Could you check a few things on this model? Use its own coordinates, in mm. A direction names the side the tool comes from. Coordinates: 2 decimals unless noted, no trailing zeros. Write each loop counter-clockwise with the first axis right and the second up, starting at its lowest first coordinate (ties: lowest second). Pieces come first, ordered by that corner, then holes. Notation, with made-up numbers: (31, -32.75) - (44, -32.75) arc R23 cw to (44, -16.75) - close; hole circle Ø1 at (8.25, 68.25). An arc over 180 degrees is marked (long way). Answer as a JSON object with one key per item and string values. Group by question number.
1) We'd pull the mould along Y, two halves only. Please class faces 5 (the cylindrical face through (-34.09, -12.08, 10.34)), 6 (the flat face through (-12.7, 0, 5)), 7 (the flat face through (13.36, 18.39, -13.38)): released by +Y, released by -Y, zero draft, split by the parting line, or undercut.
2) If we section it at B-B (x = -31.75): Write out the boundary of the cut face in (y, z).
3) If we section it at D-D (y = -19.5): Write out the boundary of the cut face in (x, z), plus the area to 3 significant figures.
4) Will these pins go through, and if not, where does the flat tip stop? pin 1 Ø1.5 at (y, z) = (-7.5, 12.5) entering from +X; pin 2 Ø15 at (x, y) = (12.5, 8.5) entering from +Z; pin 3 Ø12.5 at (y, z) = (-6, -9.5) entering from -X.
5) If we section it at C-C (z = 5): Write out the boundary of the cut face in (x, y), plus the area to 3 significant figures.
6) On a 3-axis mill with a long thin cutter (end or side, diameter ignored), from which of +Z, -Z, +X, -X, +Y, -Y can I reach the whole of each face in a straight line? I mean faces 1 (the flat face through (-22.098, 0, -7)), 2 (the cylindrical face through (-28.82, -19.858, 16.671)), 3 (the flat face through (-46, 0, -1.524)), 4 (the flat face through (29, -11.176, -13)). Say none if no direction works.
7) Please list where these lines run through material, in increasing order: line 1 along Y through (x, z) = (-31.75, 8.5); line 2 along Y through (x, z) = (38.1, -10.5); line 3 along X through (y, z) = (-12, 6).
8) If we section it at A-A (y = 0): Write out the boundary of the cut face in (x, z), plus the area to 3 significant figures.
```python
from build123d import *

# Parameters (mm, degrees)
F0_W     = 50.8
F0_H     = 38.1
F1_DEPTH = 50.8
F2_R     = 3.175
F3_DEPTH = 38.101
F4_W     = 63.5
F4_H     = 26.924
F5_DEPTH = 50.801
F6_R     = 6.35
F7_DEPTH = 11.177
F8_R     = 6.35
F9_DEPTH = 4.826


with BuildPart() as f1:
    # F0 (on Right) → F1 (new body, symmetric)
    with BuildSketch(Plane.YZ):
        Rectangle(F0_W, F0_H)
    extrude(amount=F1_DEPTH, both=True)

    # F2 (on face) → F3 (cut, through all)
    with BuildSketch(Plane.XY.offset(19.05)):
        with Locations((-31.75, -14.224)):
            Circle(F2_R)
        with Locations((-31.75, 14.224)):
            Circle(F2_R)
    extrude(amount=-F3_DEPTH, mode=Mode.SUBTRACT)

    # F4 (on face) → F5 (cut, through all)
    with BuildSketch(Plane.XZ.offset(25.4)):
        Polygon((-41.148, -1.524), (-50.8, -1.524), (-50.8, -19.05), (-22.098, -19.05), (-22.098, 6.35), (-41.148, 6.35), align=None)
        with Locations((19.05, 5.588)):
            Rectangle(F4_W, F4_H)
    extrude(amount=-F5_DEPTH, mode=Mode.SUBTRACT)

    # F6 (on face) → F7 (cut, through all)
    with BuildSketch(Plane.XY.offset(-7.874)):
        with BuildLine():
            ThreePointArc((38.1, 11.176), (49.276, 0), (38.1, -11.176))
            Line((38.1, -11.176), (20.574, -11.176))
            Line((20.574, -11.176), (6.35, -25.4))
            Line((6.35, -25.4), (50.8, -25.4))
            Line((50.8, -25.4), (50.8, 25.4))
            Line((50.8, 25.4), (6.35, 25.4))
            Line((6.35, 25.4), (20.574, 11.176))
            Line((20.574, 11.176), (24.505507, 11.176))
            Line((24.505507, 11.176), (38.1, 11.176))
        make_face()
        with Locations((38.1, 0)):
            Circle(F6_R)
    extrude(amount=-F7_DEPTH, mode=Mode.SUBTRACT)

    # F8 (on face) → F9 (cut)
    with BuildSketch(Plane.XY.offset(19.05)):
        with Locations((-31.75, 14.224)):
            Circle(F8_R)
        with Locations((-31.75, -14.224)):
            Circle(F8_R)
    extrude(amount=-F9_DEPTH, mode=Mode.SUBTRACT)


solid = f1.part
```
Here are the results:
{
 "1": {"face 5": "undercut", "face 6": "zero draft", "face 7": "released by +Y"},
 "2": {"outline": "(-25.4, 6.35) - (-17.4, 6.35) - (-17.4, 14.22) - (-20.57, 14.22) - (-20.57, 19.05) - (-25.4, 19.05) - close; (-11.05, 6.35) - (11.05, 6.35) - (11.05, 14.22) - (7.87, 14.22) - (7.87, 19.05) - (-7.87, 19.05) - (-7.87, 14.22) - (-11.05, 14.22) - close; (17.4, 6.35) - (25.4, 6.35) - (25.4, 19.05) - (20.57, 19.05) - (20.57, 14.22) - (17.4, 14.22) - close"},
 "3": {"outline": "(-50.8, -1.52) - (-41.15, -1.52) - (-41.15, 6.35) - (-22.1, 6.35) - (-22.1, -19.05) - (12.25, -19.05) - (12.25, -7.87) - (-12.7, -7.87) - (-12.7, 19.05) - (-28.22, 19.05) - (-28.22, 14.22) - (-35.28, 14.22) - (-35.28, 19.05) - (-50.8, 19.05) - close", "area": "1,040 mm²"},
 "4": {"pin 1": "stops at x = -12.7", "pin 2": "stops at z = -7.87", "pin 3": "stops at x = -22.1"},
 "5": {"outline": "(-50.8, -25.4) - (-41.15, -25.4) - (-41.15, 25.4) - (-50.8, 25.4) - close; (-22.1, -25.4) - (-12.7, -25.4) - (-12.7, 25.4) - (-22.1, 25.4) - close", "area": "968 mm²"},
 "6": {"face 1": "-Z, +Y, -Y", "face 2": "+Z", "face 3": "-Z, -X, +Y, -Y", "face 4": "+Z, -Z, +X, -Y"},
 "7": {"line 1": "y = -25.4 to -17.4, -11.05 to 11.05, 17.4 to 25.4", "line 2": "y = -11.18 to -6.35, 6.35 to 11.18", "line 3": "x = -50.8 to -41.15, -22.1 to -12.7"},
 "8": {"outline": "(-50.8, -1.52) - (-41.15, -1.52) - (-41.15, 6.35) - (-22.1, 6.35) - (-22.1, -19.05) - (31.75, -19.05) - (31.75, -7.87) - (-12.7, -7.87) - (-12.7, 19.05) - (-50.8, 19.05) - close; (44.45, -19.05) - (49.28, -19.05) - (49.28, -7.87) - (44.45, -7.87) - close", "area": "1,350 mm²"}
}
